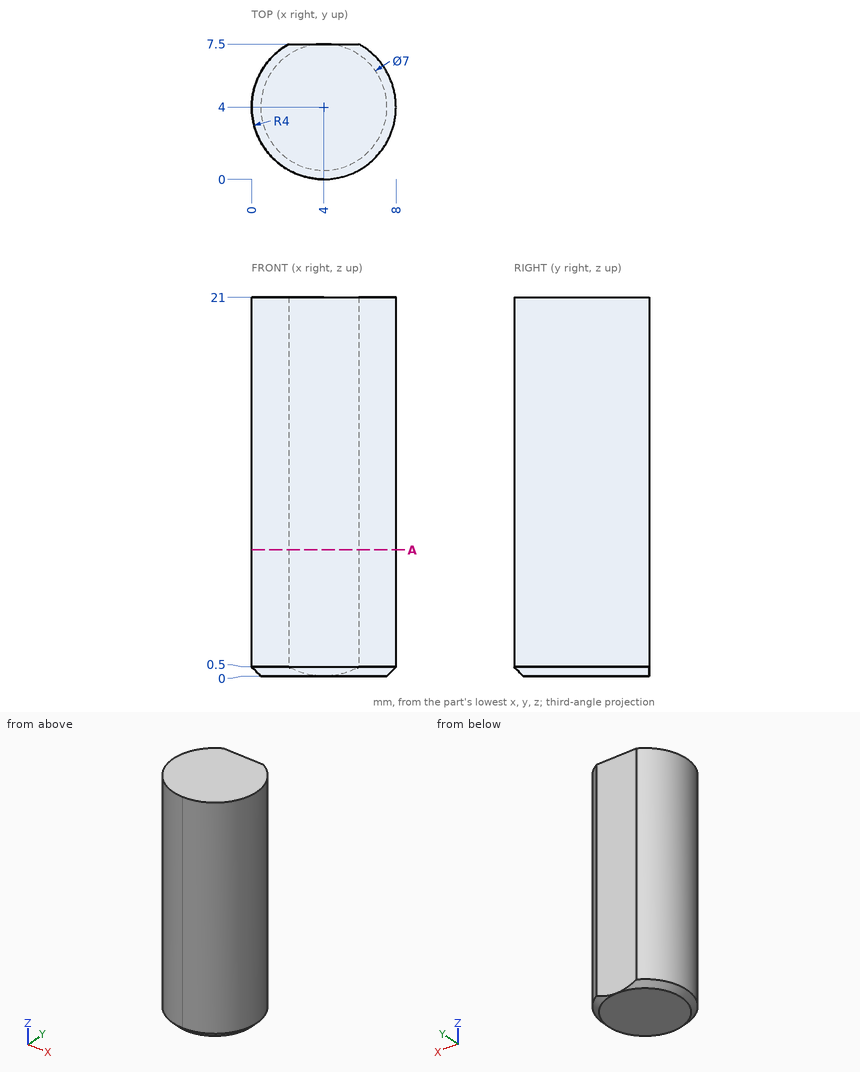
Here's the drawing with two shaded views (mm, measured from the low corner). I have some questions. Give positions to 0.01 mm unless a question says otherwise; leave off trailing zeros. Order: outer loops, then holes, each group sorted by start corner. A loop starts at its lowest first (then second) coordinate and runs counter-clockwise, first axis right, second up. Notation, with made-up numbers: (-28, 5) - (-6, 5) arc R19 cw to (-6, 33) - close; hole circle Ø9 at (31, 86.25). An arc over 180 degrees is marked (long way). Use a Markdown table: item, result. Add a question column.
Q1. Please list where these lines run through material, in increasing order: line 1 along Y through (x, z) = (7.5, 6); line 2 along Y through (x, z) = (4.5, 16.75).
Q2. If we section it at A-A on z = 7: Write out the boundary of the cut face in (x, y).
Q3. I'm going to push a flat-ended pin straight in: pin 1 (1.5 mm diameter, centred on y = 1.5, z = 13.5, fed in from -X). Where does the tip first touch, or does it pass through?
Answers follow:
| question | item | result |
|---|---|---|
| 1 | line 1 | y = 2.06 to 5.94 |
| 1 | line 2 | y = 0.03 to 7.5 |
| 2 | outline | (2.06, 7.5) arc R4 ccw to (4, 0) arc R4 ccw to (5.94, 7.5) - close |
| 3 | pin 1 | stops at x = 0.4 |
